Print and shaded views of the part. All mm, measured from the part's lowest x, y and z. A direction names the side the tool comes from. Give positions to 0.01 mm unless a question says otherwise; leave off trailing zeros. Loops run counter-clockwise (first coordinate to the right, second up) from the corner with the lowest first, then second, coordinate; pieces in that order, holes last. Notation, with made-up numbers: (-25, -9) -> (-14, -9) arc R20 cw to (-14, 25) -> close; hole circle Ø3 at (-35, -34). An arc over 180 degrees is marked (long way). Write each question's results on one line, items separated by ' | '. Start each with the question number.
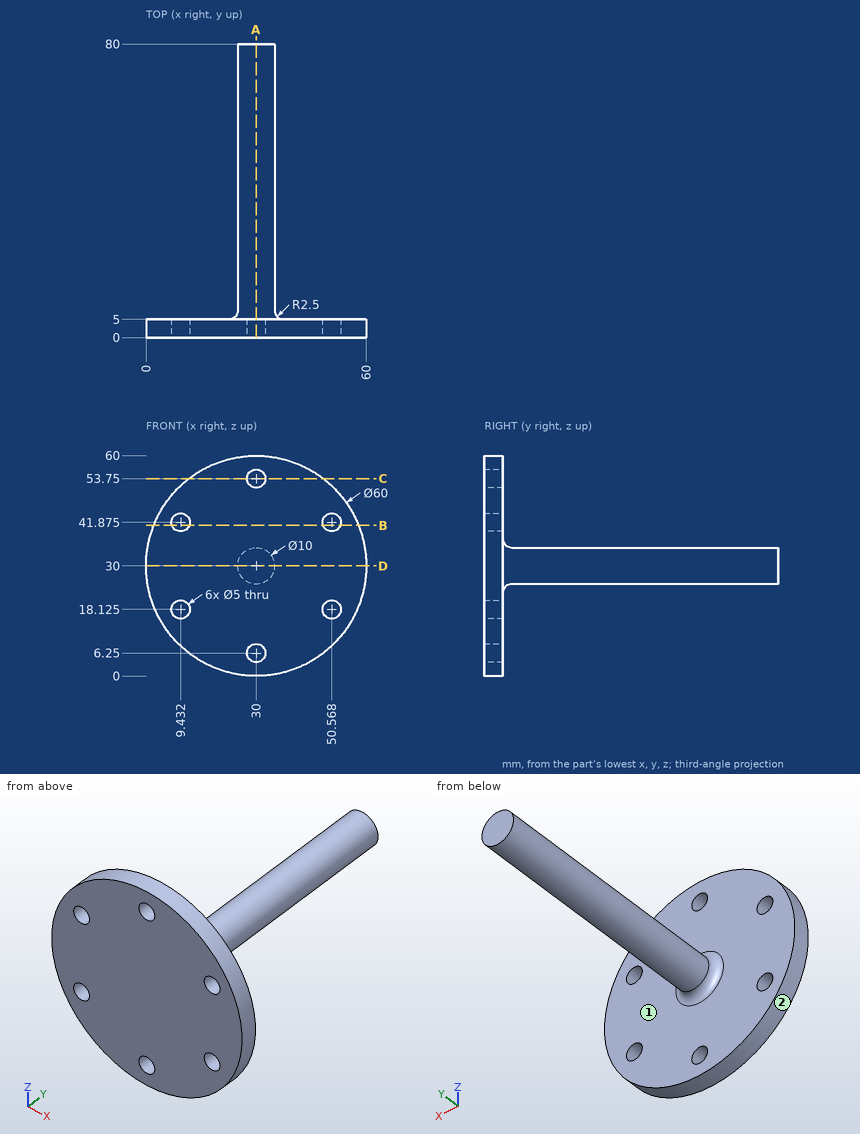
Q1. Saw through at D-D, the plane z = 30. List the corners of the cut face in (x, y), then the cut area to 3 significant figures.
Q2. Saw through at B-B, the plane z = 41. List the corners of the cut face in (x, y), then the cut area to 3 significant figures.
Q3. Wall check: L1, parallel to Y at x = 52, z = 39; L2, parallel to X at y = 1.05, z = 53.75; L3, parallel to Z at x = 34.5, y = 45. Give the ranges that are in metal, low to high.
Q4. Saw through at A-A, the plane x = 30. List the corners of the cut face in (y, z).
Q5. Drop flat-ended pins along their axis: pin 1 (1.5 mm diameter, centred on y = 65.5, z = 24, fed in from -X); pin 2 (8 mm diameter, centred on x = 9.43, z = 18.12, fed in from +Y); pin 3 (1 mm diameter, centred on y = 56, z = 32, fed in from +X). Give the stop position or say it passes through.
Q6. Which spindle directions (+Z, -Z, +X, -X, +Y, -Y) get a long thin tool onto all of the face, cutting with end or side? Do the marked faces 1 and 2. Say none if no direction does.
Q7. Saw through at C-C, the plane z = 53.75. List the corners of the cut face in (x, y), then the cut area to 3 significant figures.
Answer block:
1) outline: (0, 0) -> (60, 0) -> (60, 5) -> (37.5, 5) arc R2.5 cw to (35, 7.5) -> (35, 80) -> (25, 80) -> (25, 7.5) arc R2.5 cw to (22.5, 5) -> (0, 5) -> close | area: 1,050 mm2
2) outline: (2.09, 0) -> (7.09, 0) -> (7.09, 5) -> (2.09, 5) -> close; (11.77, 0) -> (48.23, 0) -> (48.23, 5) -> (11.77, 5) -> close; (52.91, 0) -> (57.91, 0) -> (57.91, 5) -> (52.91, 5) -> close | area: 232 mm2
3) L1: y = 0 to 5 | L2: x = 11.67 to 27.5, 32.5 to 48.33 | L3: z = 27.82 to 32.18
4) outline: (0, 0) -> (5, 0) -> (5, 3.75) -> (0, 3.75) -> close; (0, 8.75) -> (5, 8.75) -> (5, 22.5) arc R2.5 cw to (7.5, 25) -> (80, 25) -> (80, 35) -> (7.5, 35) arc R2.5 cw to (5, 37.5) -> (5, 51.25) -> (0, 51.25) -> close; (0, 56.25) -> (5, 56.25) -> (5, 60) -> (0, 60) -> close
5) pin 1: passes through | pin 2: stops at y = 5 | pin 3: stops at x = 34.77
6) face 1: +Y | face 2: +Y, -Y
7) outline: (11.67, 0) -> (27.5, 0) -> (27.5, 5) -> (11.67, 5) -> close; (32.5, 0) -> (48.33, 0) -> (48.33, 5) -> (32.5, 5) -> close | area: 158 mm2
